Check sheet for the drawn part. Datum: minimum x, y, z corner. Units: mm. A direction names the side the tool comes from. Coordinates: 2 decimals unless noted, no trailing zeros. Loops run counter-clockwise (first coordinate to the right, second up) from the corner with the lowest first, then second, coordinate; pieces in that order, holes last.
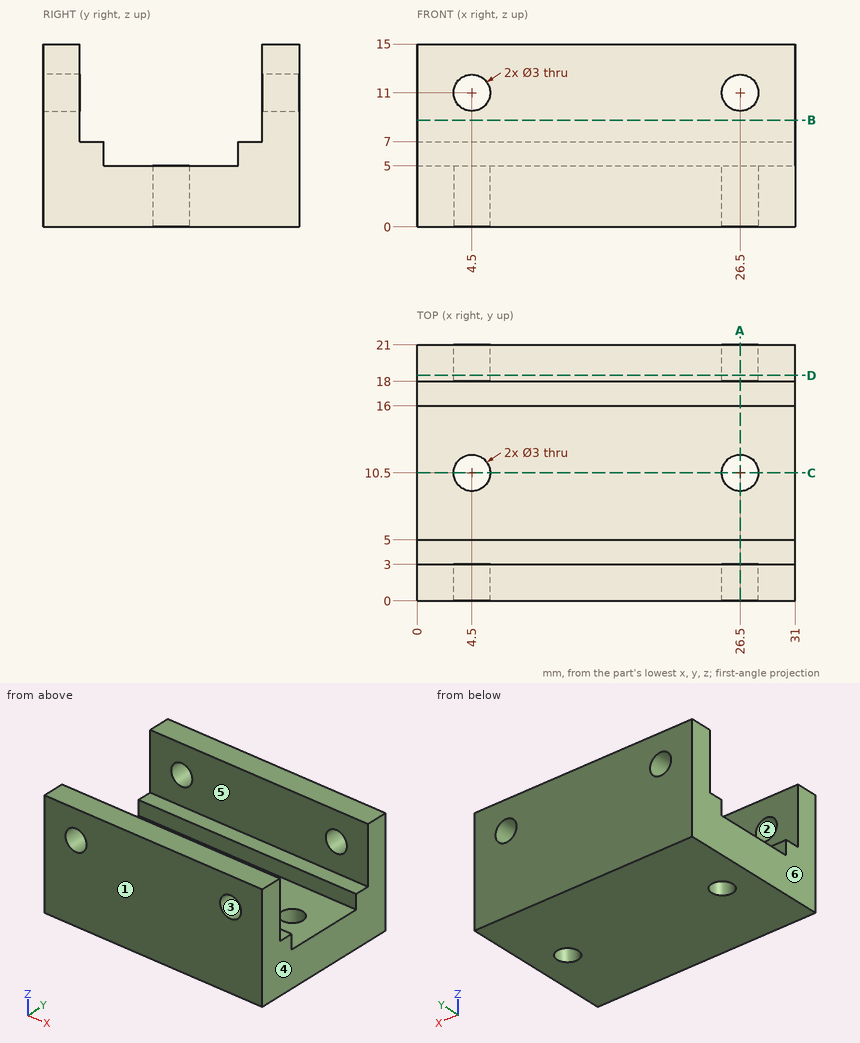
(1) Gauge pin test, flat ends, axial feed: pin 1 Ø5.5 at (x, y) = (17.5, 8) entering from +Z; pin 2 Ø0.6 at (x, y) = (16, 4.5) entering from +Z. Record the tip position at first contact, or that the pin passes through.
Findings:
pin 1: stops at z = 5
pin 2: stops at z = 7
(2) Sectioned sample at C-C on y = 10.5. Record the cut outline in (x, z), and give its area (3 significant figures).
Findings:
outline: (0, 0) - (3, 0) - (3, 5) - (0, 5) - close; (6, 0) - (25, 0) - (25, 5) - (6, 5) - close; (28, 0) - (31, 0) - (31, 5) - (28, 5) - close
area: 125 mm2
(3) Scan lines: L1, parallel to X at y = 2.4, z = 11; L2, parallel to Y at x = 12, z = 6.75; L3, parallel to Y at x = 26.5, z = 2.15. Record each from-to range of solid material in increasing order.
Findings:
L1: x = 0 to 3, 6 to 25, 28 to 31
L2: y = 0 to 5, 16 to 21
L3: y = 0 to 9, 12 to 21
(4) Draft check along X on the marked faces 1, 2, 3 and 4. Enter one of: +X half, -X half, draft (parallel to the pull), parting line (faces both ways), or undercut.
Findings:
face 1: draft
face 2: undercut
face 3: undercut
face 4: +X half
(5) Sectioned sample at A-A on x = 26.5. Record the cut outline in (y, z).
Findings:
outline: (0, 0) - (9, 0) - (9, 5) - (5, 5) - (5, 7) - (3, 7) - (3, 9.5) - (0, 9.5) - close; (0, 12.5) - (3, 12.5) - (3, 15) - (0, 15) - close; (12, 0) - (21, 0) - (21, 9.5) - (18, 9.5) - (18, 7) - (16, 7) - (16, 5) - (12, 5) - close; (18, 12.5) - (21, 12.5) - (21, 15) - (18, 15) - close
(6) Sectioned sample at B-B on z = 8.75. Record the cut outline in (x, y), and give its area (3 significant figures).
Findings:
outline: (0, 0) - (31, 0) - (31, 3) - (0, 3) - close; (0, 18) - (31, 18) - (31, 21) - (0, 21) - close
area: 186 mm2
(7) Access from +Z, -Z, +X, -X, +Y, -Y to the whole of each face (thin tool, end or side, straight path). Record for the marked faces 5 and 6.
Findings:
face 5: +Z, +X, -X
face 6: +Z, -Z, -X, +Y, -Y
(8) Sectioned sample at D-D on y = 18.5. Record the cut outline in (x, z), and give its area (3 significant figures).
Findings:
outline: (0, 0) - (31, 0) - (31, 15) - (0, 15) - close; hole circle Ø3 at (4.5, 11); hole circle Ø3 at (26.5, 11)
area: 451 mm2
